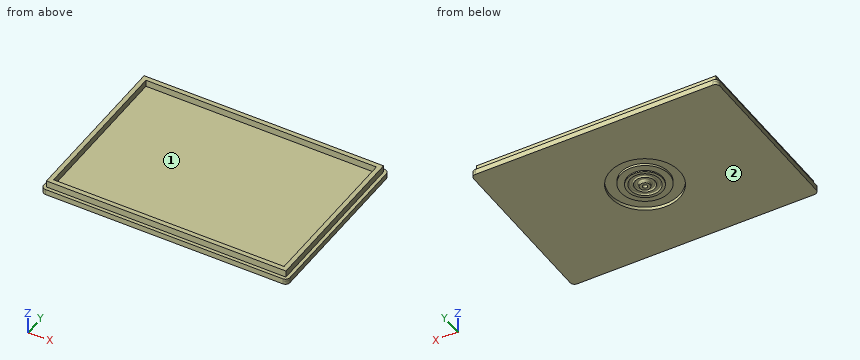
from build123d import *

# Parameters (mm, degrees)
F2_W      = 109.5
F2_H      = 76.5
F3_DEPTH  = 1
F1_W      = 106.5
F1_H      = 73.5
F4_DEPTH  = 3
F0_W      = 102.5
F0_H      = 69.5
F5_DEPTH  = 3
F6_R      = 10.8
F7_DEPTH  = 1
F8_R      = 2.25
F8_R_2    = 1
F9_DEPTH  = 2.5
F10_R     = 7.825
F10_R_2   = 6.575
F11_DEPTH = 0.6
F12_R     = 4.4225
F12_R_2   = 4.4125
F13_DEPTH = 0.6
F14_R     = 0.59999
F15_R     = 2
F16_R     = 15.5
F17_DEPTH = 1.5


# Not quite as in the source:
# - a fillet or chamfer is up to 0.001 mm smaller than in the source, because OpenCascade refuses the exact size


with BuildPart() as f3:
    # F2 (on Top) → F3 (new body)
    with BuildSketch(Plane.XY):
        Rectangle(F2_W, F2_H)
    extrude(amount=-F3_DEPTH)

    # F1 (on Top) → F4 (join)
    with BuildSketch(Plane.XY):
        Rectangle(F1_W, F1_H)
    extrude(amount=F4_DEPTH)

    # F0 (on Top) → F5 (cut, through all)
    with BuildSketch(Plane.XY):
        Rectangle(F0_W, F0_H)
    extrude(amount=F5_DEPTH, mode=Mode.SUBTRACT)

    # F6 (on face) → F7 (join)
    with BuildSketch(Plane(origin=(0, 0, -1), x_dir=(1, 0, 0), z_dir=(0, 0, -1))):
        Circle(F6_R)
    extrude(amount=F7_DEPTH)

    # F8 (on face) → F9 (join)
    with BuildSketch(Plane(origin=(0, 0, -1), x_dir=(1, 0, 0), z_dir=(0, 0, -1))):
        Circle(F8_R)
        Circle(F8_R_2, mode=Mode.SUBTRACT)
    extrude(amount=F9_DEPTH)

    # F10 (on face) → F11 (join)
    with BuildSketch(Plane(origin=(0, 0, -2), x_dir=(1, 0, 0), z_dir=(0, 0, -1))):
        Circle(F10_R)
        Circle(F10_R_2, mode=Mode.SUBTRACT)
    extrude(amount=F11_DEPTH)

    # F12 (on face) → F13 (join)
    with BuildSketch(Plane(origin=(0, 0, -2), x_dir=(1, 0, 0), z_dir=(0, 0, -1))):
        Circle(F12_R)
        Circle(F12_R_2, mode=Mode.SUBTRACT)
    extrude(amount=F13_DEPTH)

    # F14 (radius 0.6 in the source; OpenCascade refuses exactly that, so slightly less here)
    f14_edges = [f3.edges().sort_by_distance(p)[0] for p in [
        (-4.4225, 0, -2),
        (-6.575, 0, -2),
        (-2.25, 0, -2),
        (-4.4125, 0, -2),
    ]]
    fillet(f14_edges, radius=F14_R)

    # F15
    f15_edges = [f3.edges().sort_by_distance(p)[0] for p in [
        (-54.75, -38.25, -0.5),
        (54.75, -38.25, -0.5),
        (54.75, 38.25, -0.5),
        (-54.75, 38.25, -0.5),
    ]]
    fillet(f15_edges, radius=F15_R)

    # F16 (on face) → F17 (join)
    with BuildSketch(Plane(origin=(0, 0, -1), x_dir=(1, 0, 0), z_dir=(0, 0, -1))):
        with BuildLine():
            ThreePointArc((-52.75, 38.25), (-54.1642135624, 37.6642135624), (-54.75, 36.25))
            Line((-54.75, 36.25), (-54.75, -36.25))
            ThreePointArc((-54.75, -36.25), (-54.1642135624, -37.6642135624), (-52.75, -38.25))
            Line((-52.75, -38.25), (52.75, -38.25))
            ThreePointArc((52.75, -38.25), (54.1642135624, -37.6642135624), (54.75, -36.25))
            Line((54.75, -36.25), (54.75, 36.25))
            ThreePointArc((54.75, 36.25), (54.1642135624, 37.6642135624), (52.75, 38.25))
            Line((52.75, 38.25), (-52.75, 38.25))
        make_face()
        Circle(F16_R, mode=Mode.SUBTRACT)
    extrude(amount=F17_DEPTH)


solid = f3.part
Here's how the part is built. I have some questions about the finished solid (model axes, mm). Face numbers are marked on the shaded views. Round coordinates to 2 decimals unless told otherwise and drop trailing zeros. Order: outer loops, then holes, each group sorted by start corner. A loop starts at its lowest first (then second) coordinate and runs counter-clockwise, first axis right, second up. Notation, with made-up numbers: (25.25, 23.5) -> (63.25, 23.5) arc R19 ccw to (63.25, 49.5) -> close; hole circle Ø5 at (-15.75, 58). An arc over 180 degrees is marked (long way). Return JSON: item names as keys, results as strings.
Q1. If we section it at B-B on x = -35: List the corners of the cut face in (y, z) for me.
Filled sheet:
{"outline": "(-38.25, -2.5) -> (38.25, -2.5) -> (38.25, 0) -> (36.75, 0) -> (36.75, 3) -> (34.75, 3) -> (34.75, 0) -> (-34.75, 0) -> (-34.75, 3) -> (-36.75, 3) -> (-36.75, 0) -> (-38.25, 0) -> close"}
Q2. If we section it at D-D on y = -9.5: List the corners of the cut face in (x, z) for me, plus the area to 3 significant figures.
Filled sheet:
{"outline": "(-54.75, -2.5) -> (-12.25, -2.5) -> (-12.25, -1) -> (-5.14, -1) -> (-5.14, -2) -> (5.14, -2) -> (5.14, -1) -> (12.25, -1) -> (12.25, -2.5) -> (54.75, -2.5) -> (54.75, 0) -> (53.25, 0) -> (53.25, 3) -> (51.25, 3) -> (51.25, 0) -> (-51.25, 0) -> (-51.25, 3) -> (-53.25, 3) -> (-53.25, 0) -> (-54.75, 0) -> close", "area": "259 mm^2"}
Q3. If we section it at A-A on z = 2: List the corners of the cut face in (x, y) for me.
Filled sheet:
{"outline": "(-53.25, -36.75) -> (53.25, -36.75) -> (53.25, 36.75) -> (-53.25, 36.75) -> close; hole (-51.25, -34.75) -> (51.25, -34.75) -> (51.25, 34.75) -> (-51.25, 34.75) -> close"}
Q4. If we section it at C-C on y = 23: List the corners of the cut face in (x, z) for me, plus the area to 3 significant figures.
Filled sheet:
{"outline": "(-54.75, -2.5) -> (54.75, -2.5) -> (54.75, 0) -> (53.25, 0) -> (53.25, 3) -> (51.25, 3) -> (51.25, 0) -> (-51.25, 0) -> (-51.25, 3) -> (-53.25, 3) -> (-53.25, 0) -> (-54.75, 0) -> close", "area": "286 mm^2"}
Q5. I need wall thicknesses on line 1 along X through (y, z) = (-17, 1); line 2 along Y through (x, z) = (0, -1.85); line 3 along Y through (x, z) = (37, 1). Which ranges of each line are inside material? Lowest first, please. Write a range as from..to.
Filled sheet:
{"line 1": "x = -53.25..-51.25, 51.25..53.25", "line 2": "y = -38.25..-15.5, -10.8..10.8, 15.5..38.25", "line 3": "y = -36.75..-34.75, 34.75..36.75"}
Q6. For pin 1 Ø1.5 at (x, z) = (-20.5, 1.5) entering from +Y; pin 2 Ø1.6 at (x, y) = (0, 0) entering from +Z; pin 3 Ø3.5 at (x, z) = (-5, 2) entering from -Y; pin 4 Ø3.5 at (y, z) = (-10.5, 1) entering from -X, each with a flat end and sliding along its axis, tell me the tip position at first contact or that it passes through.
Filled sheet:
{"pin 1": "stops at y = 36.75", "pin 2": "stops at z = 0", "pin 3": "stops at y = -36.75", "pin 4": "stops at x = -54.75"}
Q7. If we mould it in two halves opening along Y, with no side actions, what happens to the marked faces 1 and 2? For each: released by +Y, released by -Y, zero draft, split by the parting line, or undercut.
Filled sheet:
{"face 1": "undercut", "face 2": "zero draft"}
